from build123d import *

# Parameters (mm, degrees)
BOSS_EXTRUDE1_DEPTH = 3
CUT_EXTRUDE3_DEPTH  = 3


with BuildPart() as part:
    # Sketch1 → Boss-Extrude1 (new body)
    with BuildSketch(Plane.XY):
        Polygon((68.5, 46), (-68.5, 46), (-68.5, 42.5), (-72, 42.5), (-72, 3.5), (-68.5, 3.5), (-68.5, 0), (68.5, 0), (68.5, 3.5), (72, 3.5), (72, 42.5), (68.5, 42.5), align=None)
    extrude(amount=BOSS_EXTRUDE1_DEPTH)

    # Sketch2 → Cut-Extrude3 (cut)
    with BuildSketch(Plane.XY.offset(3)):
        with BuildLine():
            Line((68.5, 5.5), (68.5, 40.5))
            ThreePointArc((68.5, 40.5), (67.914213562, 41.914213562), (66.5, 42.5))
            Line((66.5, 42.5), (-66.5, 42.5))
            ThreePointArc((-66.5, 42.5), (-67.914213562, 41.914213562), (-68.5, 40.5))
            Line((-68.5, 40.5), (-68.5, 5.5))
            ThreePointArc((-68.5, 5.5), (-67.914213562, 4.085786438), (-66.5, 3.5))
            Line((-66.5, 3.5), (66.5, 3.5))
            ThreePointArc((66.5, 3.5), (67.914213562, 4.085786438), (68.5, 5.5))
        make_face()
    extrude(amount=-CUT_EXTRUDE3_DEPTH, mode=Mode.SUBTRACT)


solid = part.part
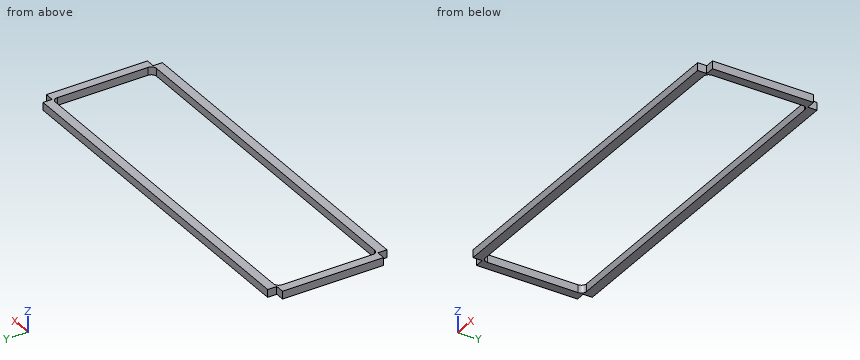
Input: part model. Units: mm. Frame: model coordinates. Coordinates: 2 decimals unless noted, no trailing zeros. Loops run counter-clockwise (first coordinate to the right, second up) from the corner with the lowest first, then second, coordinate; pieces in that order, holes last.
(1) Section B-B on y = 9. Return the cut outline in (x, z).
(2) Section C-C on z = 1.1. Return the cut outline in (x, y), then the cut area to 3 significant figures.
(3) Material intervals for probe 1 along Y at (x, z) = (-46, 1.8); probe 2 along X at (y, z) = (28, 2.5); probe 3 along X at (y, z) = (43.5, 1), sorted ascending.
(4) First-contact query: pin 1 Ø0.9 at (x, z) = (-70, 1) entering from -Y; pin 2 Ø0.9 at (y, z) = (44.5, 1.5) entering from -X; pin 3 Ø1.5 at (y, z) = (1.5, 1) entering from +X. Flat tips, straight axial feed; report the tip coordinate or a pass-through.
(5) Section A-A on x = 45.5. Return the cut outline in (y, z), then the cut area to 3 significant figures.
Data:
1. outline: (-72, 0) - (-68.5, 0) - (-68.5, 3) - (-72, 3) - close; (68.5, 0) - (72, 0) - (72, 3) - (68.5, 3) - close
2. outline: (-72, 3.5) - (-68.5, 3.5) - (-68.5, 0) - (68.5, 0) - (68.5, 3.5) - (72, 3.5) - (72, 42.5) - (68.5, 42.5) - (68.5, 46) - (-68.5, 46) - (-68.5, 42.5) - (-72, 42.5) - close; hole (-68.5, 5.5) arc R2 ccw to (-66.5, 3.5) - (66.5, 3.5) arc R2 ccw to (68.5, 5.5) - (68.5, 40.5) arc R2 ccw to (66.5, 42.5) - (-66.5, 42.5) arc R2 ccw to (-68.5, 40.5) - close
2. area: 1,240 mm2
3. probe 1: y = 0 to 3.5, 42.5 to 46
3. probe 2: x = -72 to -68.5, 68.5 to 72
3. probe 3: x = -68.5 to 68.5
4. pin 1: stops at y = 3.5
4. pin 2: stops at x = -68.5
4. pin 3: stops at x = 68.5
5. outline: (0, 0) - (3.5, 0) - (3.5, 3) - (0, 3) - close; (42.5, 0) - (46, 0) - (46, 3) - (42.5, 3) - close
5. area: 21.0 mm2
